Build history of the part. All positions in model axes, mm. A direction names the side the tool comes from. Round coordinates to 2 decimals unless told otherwise and drop trailing zeros. Order: outer loops, then holes, each group sorted by start corner. A loop starts at its lowest first (then second) coordinate and runs counter-clockwise, first axis right, second up. Notation, with made-up numbers: (-9, 17) -> (3, 17) arc R22 ccw to (3, 45) -> close; hole circle Ø1 at (67.25, 74). An arc over 180 degrees is marked (long way). Use a Markdown table: item, result. Add a question column.
Item 1: Two-plate mould, pull along Z, no slides. Class faces 1 (the face through (-2, -2, 1)), 2 (the face through (-5.311, 2.504, -1.305)), 3 (the face through (-2, 3.687, 0)): released by +Z, released by -Z, zero draft, split by the parting line, or undercut.
Item 2: Slice it at A-A, the plane y = -28.5. Give the cut face in (x, z).
Item 3: 3-axis set-ups, long thin cutter, end or side, ignore diameter. For faces 4 (the face through (-4.64, -0.813, 3.31)), 5 (the face through (-2.23, 1.257, -4.502)), 6 (the face through (-3.832, 2.504, 1.305)), 7 (the face through (-2.826, -27.005, 0.724)): which of +Z, -Z, +X, -X, +Y, -Y reach the whole face in a straight line?
Item 4: Pin check, flat tips, straight feed: pin 1 (3.5 mm diameter, centred on x = -4.5, z = 0, fed in from +Y); pin 2 (1.5 mm diameter, centred on x = -3.5, y = -10.5, fed in from -Z); pin 3 (4 mm diameter, centred on y = -19, z = 3.5, fed in from +X); pin 4 (2 mm diameter, centred on x = -8, y = -4, fed in from +Z). Stop position of each tip, or through.
Item 5: Probe L1, parallel to Y at x = -2.75, z = 3; L2, parallel to Y at x = -6.75, z = -1; L3, parallel to X at y = -29.5, z = 0.25. List the from-to ranges inside material, lowest first.
Autodesk Inventor part; units mm, degrees
ref_plane "YZ Plane" through (0, 0, 0) normal (1, 0, 0) x (0, 1, 0)
ref_plane "XZ Plane" through (0, 0, 0) normal (0, 1, 0) x (-1, 0, 0)
ref_plane "XY Plane" through (0, 0, 0) normal (0, 0, 1) x (1, 0, 0)
sketch "Sketch1" plane through (0, 0, 0) normal (0, 0, 1) x (1, 0, 0)
  line L0 (-4.5718, -2.6632) -> (-7.5718, -2.6632)
  line L1 (-7.5718, -2.6632) -> (-7.5718, -25.8132)
  line L2 (-7.5718, -25.8132) -> (-4.5718, -25.8132)
  line L3 (-4.5718, -25.8132) -> (-4.5718, -2.6632)
  dimension "d1" = 23.15
  dimension "d2" = 3
revolve "Shoulder" add sketch "Sketch1" angle 360 about axis through (-4.5718, -25.8132, 0) along (0, 1, 0)
sketch "Sketch2" plane through (-4.5718, -2.6632, 0) normal (0, 1, 0) x (1, 0, 0)
  circle A0 centre (0, 0) radius 3
  circle A1 centre (0, 0) radius 2.76
  dimension "d3" = 5.52
extrude "Shoulder_neck" add sketch "Sketch2" along normal blind 1.85 contours A1
sketch "Sketch3" plane through (-4.5718, -0.8132, 0) normal (0, 1, 0) x (1, 0, 0)
  circle A0 centre (0, 0) radius 2.76
  circle A1 centre (0, 0) radius 5.075
  dimension "d6" = 10.15
extrude "Head" add sketch "Sketch3" along normal blind 4.5 contours A0 | A1
sketch "Sketch4" plane through (-4.5718, -25.8132, 0) normal (0, -1, 0) x (1, 0, 0)
  circle A0 centre (0, 0) radius 3
  circle A1 centre (0, 0) radius 1.89
  dimension "d9" = 3.78
extrude "Thread_neck" add sketch "Sketch4" along normal blind 1.8 contours A1
sketch "Sketch5" plane through (-4.5718, -27.6132, 0) normal (0, -1, 0) x (1, 0, 0)
  circle A0 centre (0, 0) radius 1.89
  circle A1 centre (0, 0) radius 2.5
  dimension "d12" = 5
extrude "Thread_shoulder" add sketch "Sketch5" along normal blind 7.7 contours A0 | A1
sketch "Sketch6" plane through (-4.5718, 3.6868, 0) normal (0, 1, 0) x (1, 0, 0)
  circle A0 centre (0, 0) radius 5.075
  circle A1 centre (0, 0) radius 1.5 construction
  line L0 (-1.5, 0.866) -> (-1.5, -0.866)
  line L1 (-1.5, -0.866) -> (0, -1.7321)
  line L2 (0, -1.7321) -> (1.5, -0.866)
  line L3 (1.5, -0.866) -> (1.5, 0.866)
  line L4 (1.5, 0.866) -> (0, 1.7321)
  line L5 (0, 1.7321) -> (-1.5, 0.866)
  dimension "d15" = 3
extrude "Hex" cut sketch "Sketch6" against normal blind 2.4 contours L5 L4 L3 L2 L1 L0
chamfer "Chamfer1" distance 0.24 angle 30 1 edges at (-1.5718, -2.6632, 0) measured on face at (-7.436, -2.6632, -0.4595)
fillet "Fillet1" radius 0.4 1 edges at (-7.3318, -0.8132, 0)
chamfer "Chamfer2" distance 0.3 angle 30 1 edges at (-9.6468, 3.6868, 0) measured on face at (0.4867, 2.1868, 0.4084)
chamfer "Chamfer3" distance 0.4 angle 30 1 edges at (-7.0718, -35.3132, 0) measured on face at (-3.3106, -35.3132, -0.6619)
fillet "Fillet2" radius 0.6 1 edges at (-6.4618, -25.8132, 0)
chamfer "Chamfer7" distance 0.61 angle 30 1 edges at (-7.0718, -27.6132, 0) measured on face at (-2.3177, -27.6132, -0.3502)
thread "Thread"
equation "\"d1\" = Shoulder_length - Shoulder_neck_length"
equation "\"d2\" = 0.5 * Shoulder_diameter"
equation "\"d3\" = Shoulder_neck_dia"
equation "\"d4\" = Shoulder_neck_length"
equation "\"d6\" = Head_diameter"
equation "\"d7\" = Head_height"
equation "\"d9\" = Thread_neck_dia"
equation "\"d10\" = Thread_neck_length"
equation "\"d12\" = Thread_diameter"
equation "\"d13\" = Thread_length - Thread_neck_length"
equation "\"d15\" = Hex_size"
equation "\"d16\" = Hex_length"
equation "\"d18\" = -0.5 * Shoulder_neck_dia + 0.5 * Shoulder_diameter"
equation "\"d64\" = -0.5 * Shoulder_neck_dia + 0.5 * Shoulder_diameter"
equation "\"d21\" = 0.1 * Hex_size"
equation "\"d65\" = 0.1 * Hex_size"
equation "\"d23\" = 0.5 * Thread_pitch"
equation "\"d66\" = 0.5 * Thread_pitch"
equation "\"d25\" = Thread_neck_radius"
equation "\"d60\" = -0.5 * Thread_neck_dia + 0.5 * Thread_diameter"
equation "\"d67\" = -0.5 * Thread_neck_dia + 0.5 * Thread_diameter"
equation "\"Shoulder_diameter\" = 6"
equation "\"Shoulder_length\" = 25"
equation "\"Shoulder_neck_dia\" = 5.52"
equation "\"Thread_diameter\" = 5"
equation "\"Thread_length\" = 9.5"
equation "\"Head_diameter\" = 10.15"
equation "\"Head_height\" = 4.5"
equation "\"Thread_neck_dia\" = 3.78"
equation "\"Hex_size\" = 3"
equation "\"Hex_length\" = 2.4"
equation "\"Thread_pitch\" = 0.8"
equation "\"Shoulder_neck_length\" = 1.85"
equation "\"Thread_neck_length\" = 1.8"
equation "\"Thread_neck_radius\" = 0.6"
properties part number "SCREW,SHOULDER,P,12.9,M6X25MM" material "Steel, High Strength Low Alloy"
Check sheet entries:
| question | item | result |
|---|---|---|
| 1 | face 1 | split by the parting line |
| 1 | face 2 | undercut |
| 1 | face 3 | zero draft |
| 2 | outline | circle Ø5 at (-4.57, 0) |
| 3 | face 4 | -Y |
| 3 | face 5 | +Y, -Y |
| 3 | face 6 | +Y |
| 3 | face 7 | none |
| 4 | pin 1 | y = 3.69 |
| 4 | pin 2 | z = -2.98 |
| 4 | pin 3 | x = -1.97 |
| 4 | pin 4 | z = 1.76 |
| 5 | L1 | -0.81 to 3.69 |
| 5 | L2 | -35.14 to -27.91, -25.82 to 3.69 |
| 5 | L3 | -7.06 to -2.08 |
